from build123d import *

# Parameters (mm, degrees)
BOX003_W            = 8
BOX003_H            = 6
BOX003_DEPTH        = 3
FILLET003_R         = 1
BOX004_W            = 25.5
BOX004_H            = 5
BOX004_DEPTH        = 9
CYLINDER_R          = 1.5
CYLINDER_DEPTH      = 3.5
CYLINDER_ROLL_ANGLE = 90
SKETCH_W            = 32
SKETCH_H            = 42
PAD_DEPTH           = 25
SKETCH001_W         = 29
SKETCH001_H         = 39
POCKET_DEPTH        = 23.5
FILLET001_R         = 1


with BuildPart() as fillet003:
    # Box003 → Box003 (new body)
    with BuildSketch(Plane(origin=(26, -16, 6.5), x_dir=(1, 0, 0), z_dir=(0, 0, 1))):
        with Locations((4, 3)):
            Rectangle(BOX003_W, BOX003_H)
    extrude(amount=BOX003_DEPTH)

    # Fillet003
    fillet003_edges = [fillet003.edges().sort_by_distance(p)[0] for p in [
        (26, -16, 8),
        (26, -13, 9.5),
        (26, -10, 8),
        (26, -13, 6.5),
        (34, -16, 8),
        (34, -13, 9.5),
        (34, -10, 8),
        (34, -13, 6.5),
        (30, -16, 6.5),
        (30, -16, 9.5),
        (30, -10, 6.5),
        (30, -10, 9.5),
    ]]
    fillet(fillet003_edges, radius=FILLET003_R)


with BuildPart() as fillet003_1:
    # Fillet003 placement: moved
    add(fillet003.part.moved(Location((0, -1, 0))))


with BuildPart() as cubo001:
    # Box004 → Box004 (new body)
    with BuildSketch(Plane(origin=(17, 24, 12.5), x_dir=(1, 0, 0), z_dir=(0, 0, 1))):
        with Locations((12.75, 2.5)):
            Rectangle(BOX004_W, BOX004_H)
    extrude(amount=BOX004_DEPTH)


with BuildPart() as holes:
    # Cylinder → Cylinder (new body)
    with BuildSketch(Plane.XY):
        Circle(CYLINDER_R)
    extrude(amount=CYLINDER_DEPTH)


with BuildPart() as holes_1:
    # Cylinder roll: moved
    add(holes.part.rotate(Axis((0, 0, 0), (1, 0, 0)), CYLINDER_ROLL_ANGLE))


with BuildPart() as holes_2:
    # Cylinder placement: moved
    add(holes_1.part.moved(Location((29.9, -12.65, 17))))

    # Fusion001: union Fillet003, Cubo001
    add(fillet003_1.part)
    add(cubo001.part)


with BuildPart() as cabinet_drilled:
    # Sketch → Pad (new body)
    with BuildSketch(Plane.XY):
        with Locations((29.906403, 6.669162)):
            Rectangle(SKETCH_W, SKETCH_H)
    extrude(amount=PAD_DEPTH)

    # Sketch001 (on Face6 of Pad) → Pocket (cut)
    with BuildSketch(Plane.XY.offset(25)):
        with Locations((29.906403, 6.669162)):
            Rectangle(SKETCH001_W, SKETCH001_H)
    extrude(amount=-POCKET_DEPTH, mode=Mode.SUBTRACT)

    # Fillet001
    fillet001_edges = [cabinet_drilled.edges().sort_by_distance(p)[0] for p in [
        (13.906403, 27.669162, 12.5),
        (45.906403, 27.669162, 12.5),
        (29.906403, 27.669162, 0),
        (13.906403, -14.330838, 12.5),
        (13.906403, 6.669162, 0),
        (45.906403, -14.330838, 12.5),
        (45.906403, 6.669162, 0),
        (29.906403, -14.330838, 0),
    ]]
    fillet(fillet001_edges, radius=FILLET001_R)


with BuildPart() as cabinet_drilled_1:
    # Fillet001 placement: moved
    add(cabinet_drilled.part.moved(Location((-0.005501, -0.803173, 0))))

    # Cut: cut Holes
    add(holes_2.part, mode=Mode.SUBTRACT)


solid = cabinet_drilled_1.part
For this review, take the finished solid that the model builds, in its own axes (mm). A direction names the side the tool comes from. Give positions to 0.01 mm unless a question says otherwise; leave off trailing zeros. Order: outer loops, then holes, each group sorted by start corner. A loop starts at its lowest first (then second) coordinate and runs counter-clockwise, first axis right, second up. Notation, with made-up numbers: M 47,19.5 L 75,19.5 A22 cw 75,39.5 Z; hole C 42,9 d10. An arc over 180 degrees is marked long. Answer in a Markdown table with one row per item. Add a question column.
(1) For pin 1 (5 mm diameter, centred on x = 29.9, z = 17, fed in from +Y); pin 2 (14.5 mm diameter, centred on x = 33, y = 10, fed in from +Z); pin 3 (0.8 mm diameter, centred on x = 36, y = 26.5, fed in from -Z), all flat-tipped, find the tip position at first contact; note any pin that passes through.
(2) Consider section A-A on x = 29.9. State the section outline as (y, z) points, and give its area (3 significant figures).
(3) Consider section C-C on x = 20. State the section outline as (y, z) points, and give its area (3 significant figures).
(4) Consider section B-B on z = 17. State the section outline as (x, y) points, and give its area (3 significant figures).
(5) Consider section D-D on z = 13.5. State the section outline as (x, y) points, and give its area (3 significant figures).
(6) For faces 5 (the face through (30, 26, 21.5)), 6 (the face through (30, -13.634, 13)), 7 (the face through (30.11, 26.58, 0.3)), 8 (the face through (14.186, 6.146, 0.301)), 9 (the face through (34, -14, 8)), list the 3-axis set-ups (+Z, -Z, +X, -X, +Y, -Y) from which the entire face can be reached by the end or side of a thin tool; tool diameter is ignored.
(7) Mouldability with a two-part tool opening along X and no side actions: class faces 1 (the face through (26, -14, 8)), 2 (the face through (45.6, -14.85, 13.17)), 3 (the face through (31.33, -14.37, 17.45)), 4 (the face through (14.186, -14.833, 13.168)) as +X half, -X half, draft (parallel to the pull), parting line (faces both ways), or undercut.
(8) Wall thickness on probe 1 along Z at (x, y) = (29.9, -14); probe 2 along Y at (x, z) = (19.5, 10.5); probe 3 along X at (y, z) = (4.5, 23): over which ranges is each line inside the solid? List them lowest first. Write a range as [from, to].
Evaluation:
| question | item | result |
|---|---|---|
| 1 | pin 1 | stops at y = -13.63 |
| 1 | pin 2 | stops at z = 1.5 |
| 1 | pin 3 | stops at z = 0.03 |
| 2 | outline | M -15.13,1 A1 ccw -14.13,0 L 25.87,0 A1 ccw 26.87,1 L 26.87,12.5 L 25.37,12.5 L 25.37,1.5 L -13.63,1.5 L -13.63,6.5 L -15.13,6.5 Z; M -15.13,9.5 L -13.63,9.5 L -13.63,15.5 L -15.13,15.5 Z; M -15.13,18.5 L -13.63,18.5 L -13.63,25 L -15.13,25 Z; M 25.37,21.5 L 26.87,21.5 L 26.87,25 L 25.37,25 Z |
| 2 | area | 111 mm^2 |
| 3 | outline | M -15.13,1 A1 ccw -14.13,0 L 25.87,0 A1 ccw 26.87,1 L 26.87,12.5 L 25.37,12.5 L 25.37,1.5 L -13.63,1.5 L -13.63,25 L -15.13,25 Z; M 25.37,21.5 L 26.87,21.5 L 26.87,25 L 25.37,25 Z |
| 3 | area | 120 mm^2 |
| 4 | outline | M 13.9,-14.13 A1 ccw 14.9,-15.13 L 28.4,-15.13 L 28.4,-13.63 L 15.4,-13.63 L 15.4,25.37 L 17,25.37 L 17,26.87 L 14.9,26.87 A1 ccw 13.9,25.87 Z; M 31.4,-15.13 L 44.9,-15.13 A1 ccw 45.9,-14.13 L 45.9,25.87 A1 ccw 44.9,26.87 L 42.5,26.87 L 42.5,25.37 L 44.4,25.37 L 44.4,-13.63 L 31.4,-13.63 Z |
| 4 | area | 169 mm^2 |
| 5 | outline | M 13.9,-14.13 A1 ccw 14.9,-15.13 L 44.9,-15.13 A1 ccw 45.9,-14.13 L 45.9,25.87 A1 ccw 44.9,26.87 L 42.5,26.87 L 42.5,25.37 L 44.4,25.37 L 44.4,-13.63 L 15.4,-13.63 L 15.4,25.37 L 17,25.37 L 17,26.87 L 14.9,26.87 A1 ccw 13.9,25.87 Z |
| 5 | area | 174 mm^2 |
| 6 | face 5 | +Y |
| 6 | face 6 | +Z |
| 6 | face 7 | -Z, +X, -X, +Y |
| 6 | face 8 | -Z, -X, +Y, -Y |
| 6 | face 9 | -Y |
| 7 | face 1 | undercut |
| 7 | face 2 | +X half |
| 7 | face 3 | undercut |
| 7 | face 4 | -X half |
| 8 | probe 1 | z = [0, 6.5], [9.5, 15.5], [18.5, 25] |
| 8 | probe 2 | y = [-15.13, -13.63], [25.37, 26.87] |
| 8 | probe 3 | x = [13.9, 15.4], [44.4, 45.9] |
